from build123d import *

# Parameters (mm, degrees)
F0_W     = 88.9
F0_H     = 88.9
F1_DEPTH = 203.2
F3_DEPTH = 88.9


with BuildPart() as f1:
    # F0 (on Top) → F1 (new body)
    with BuildSketch(Plane.XY):
        with Locations((2.694333, -0.491857)):
            Rectangle(F0_W, F0_H)
    extrude(amount=F1_DEPTH)

    # F2 (on face) → F3 (cut)
    with BuildSketch(Plane.XY.offset(203.2)):
        Polygon((9.044333, 43.958143), (-41.755667, 43.958143), (-41.755667, 5.858143), (9.044333, 5.858143), (9.044333, -44.941857), (47.144333, -44.941857), (47.144333, 5.858143), (47.144333, 43.958143), align=None)
    extrude(amount=-F3_DEPTH, mode=Mode.SUBTRACT)


solid = f1.part
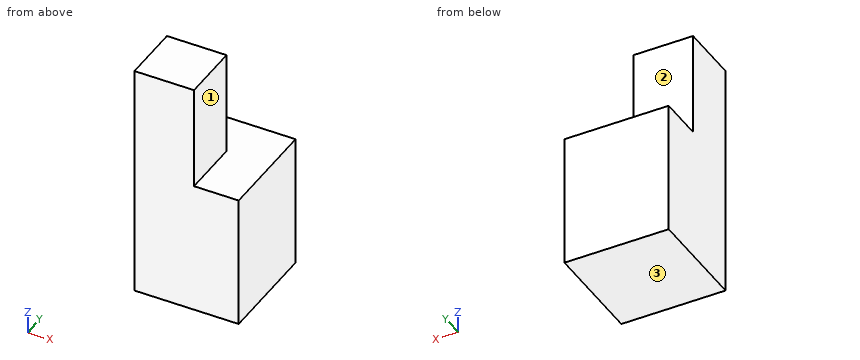
For this review, take the finished solid that the model builds, in its own axes (mm). Face numbers are marked on the shaded views. A direction names the side the tool comes from. Round coordinates to 2 decimals unless told otherwise and drop trailing zeros. Loops run counter-clockwise (first coordinate to the right, second up) from the corner with the lowest first, then second, coordinate; pieces in that order, holes last. Notation, with made-up numbers: (10.5, 37.25) - (43.5, 37.25) arc R34 cw to (43.5, 68.25) - close; hole circle Ø11 at (30.25, 21.5). An arc over 180 degrees is marked (long way). Answer as CSV lines item,"result".
(1) Consider section D-D on y = -16. Give the boundary of the cut face in (x, z).
Checked values:
outline,"(-41.76, 0) - (47.14, 0) - (47.14, 114.3) - (9.04, 114.3) - (9.04, 203.2) - (-41.76, 203.2) - close"
(2) Consider section C-C on y = 37. Give the boundary of the cut face in (x, z).
Checked values:
outline,"(-41.76, 0) - (47.14, 0) - (47.14, 114.3) - (-41.76, 114.3) - close"
(3) Tool access review of the marked faces 1, 2 and 3: name each direction out of +Z, -Z, +X, -X, +Y, -Y from which nothing blocks a thin tool from reaching the whole face with its end or side.
Checked values:
face 1,"+Z, +X, +Y, -Y"
face 2,"+Z, +X, -X, +Y"
face 3,"-Z, +X, -X, +Y, -Y"
(4) Insertion check: P1, Ø4, axis at x = -3, z = 165, coming from the +Y side; P2, Ø1, axis at y = -32, z = 182.5, coming from the +X side. Each pin has a flat end and moves straight along its axis. Give the tip position at first contact, or say it passes through.
Checked values:
P1,"stops at y = 5.86"
P2,"stops at x = 9.04"
(5) Consider section A-A on x = 5.5. Give the boundary of the cut face in (y, z), then the cut area to 3 significant figures.
Checked values:
outline,"(-44.94, 0) - (43.96, 0) - (43.96, 114.3) - (5.86, 114.3) - (5.86, 203.2) - (-44.94, 203.2) - close"
area,"14,700 mm2"
(6) Wall thickness on line 1 (X direction, y = -18.5, z = 157.5); line 2 (Y direction, x = -19, z = 195); line 3 (Z direction, x = 25, y = -19): over which ranges is each line inside the solid? List them lowest first.
Checked values:
line 1,"x = -41.76 to 9.04"
line 2,"y = -44.94 to 5.86"
line 3,"z = 0 to 114.3"
(7) Consider section B-B on z = 158. Give the boundary of the cut face in (x, y).
Checked values:
outline,"(-41.76, -44.94) - (9.04, -44.94) - (9.04, 5.86) - (-41.76, 5.86) - close"
